```python
from build123d import *

# Parameters (mm, degrees)
F1_DEPTH = 3
F2_W     = 90
F2_H     = 55
F3_DEPTH = 24
F4_R     = 1.25
F5_DEPTH = 10
F6_W     = 13
F6_H     = 65
F7_DEPTH = 9
F8_R     = 3


with BuildPart() as f1:
    # F0 (on Top) → F1 (new body)
    with BuildSketch(Plane.XY):
        with BuildLine():
            ThreePointArc((0, 5), (1.464466, 1.464466), (5, 0))
            Line((5, 0), (99, 0))
            ThreePointArc((99, 0), (102.535534, 1.464466), (104, 5))
            Line((104, 5), (104, 60))
            ThreePointArc((104, 60), (102.535534, 63.535534), (99, 65))
            Line((99, 65), (5, 65))
            ThreePointArc((5, 65), (1.464466, 63.535534), (0, 60))
            Line((0, 60), (0, 5))
        make_face()
    extrude(amount=F1_DEPTH)

    # F2 (on face) → F3 (join)
    with BuildSketch(Plane.XY.offset(3)):
        with BuildLine():
            Line((0, 60), (0, 5))
            ThreePointArc((0, 5), (1.464466, 1.464466), (5, 0))
            Line((5, 0), (99, 0))
            ThreePointArc((99, 0), (102.535534, 1.464466), (104, 5))
            Line((104, 5), (104, 60))
            ThreePointArc((104, 60), (102.535534, 63.535534), (99, 65))
            Line((99, 65), (5, 65))
            ThreePointArc((5, 65), (1.464466, 63.535534), (0, 60))
        make_face()
        with Locations((52, 32.5)):
            Rectangle(F2_W, F2_H, mode=Mode.SUBTRACT)
    extrude(amount=F3_DEPTH)

    # F4 (on face) → F5 (cut)
    with BuildSketch(Plane.XY.offset(27)):
        with Locations((3.5, 10)):
            Circle(F4_R)
        with Locations((100.5, 55)):
            Circle(F4_R)
        with Locations((100.5, 10)):
            Circle(F4_R)
        with Locations((3.5, 55)):
            Circle(F4_R)
    extrude(amount=-F5_DEPTH, mode=Mode.SUBTRACT)

    # F6 (on face) → F7 (cut)
    with BuildSketch(Plane.XY.offset(27)):
        with Locations((19.5, 32.5)):
            Rectangle(F6_W, F6_H)
    extrude(amount=-F7_DEPTH, mode=Mode.SUBTRACT)

    # F8
    f8_edges = [f1.edges().sort_by_distance(p)[0] for p in [
        (26, 2.5, 18),
        (26, 62.5, 18),
        (13, 62.5, 18),
        (13, 2.5, 18),
    ]]
    fillet(f8_edges, radius=F8_R)


solid = f1.part
```
Part model, mm, in its own coordinate system. A direction names the side the tool comes from. Round coordinates to 2 decimals unless told otherwise and drop trailing zeros. Order: outer loops, then holes, each group sorted by start corner. A loop starts at its lowest first (then second) coordinate and runs counter-clockwise, first axis right, second up. Notation, with made-up numbers: M 44,-21 L 63,-21 A18 ccw 63,1 Z; hole C 53,47.25 d4. An arc over 180 degrees is marked long. Answer in a Markdown table with one row per item. Add a question column.
Q1. Cut at A-A on z = 7.25. Give the cut face in (x, y), and give its area (3 significant figures).
Q2. Wall check: L1, parallel to Y at x = 67, z = 17.5; L2, parallel to X at y = 54, z = 8; L3, parallel to Y at x = 100.5, z = 24. Give the ranges that are in metal, low to high. Write a range as from..to.
Q3. Cut at C-C on x = 88. Give the cut face in (y, z).
Q4. 3-axis set-ups, long thin cutter, end or side, ignore diameter. For faces 5 (the face through (101.69, 10.38, 22.07)), 6 (the face through (51, 0, 13)), 7 (the face through (19, 3, 18)): which of +Z, -Z, +X, -X, +Y, -Y reach the whole face in a straight line?
Q5. Cut at D-D on y = 55. Give the cut face in (x, z), and give its area (3 significant figures).
Q6. Cut at B-B on y = 20. Give the cut face in (x, z), and give its area (3 significant figures).
Q7. Pin check, flat tips, straight feed: pin 1 (2.5 mm diameter, centred on x = 21, y = 1.5, fed in from +Z); pin 2 (5 mm diameter, centred on x = 57, y = 42, fed in from +Z); pin 3 (1.5 mm diameter, centred on y = 1.5, z = 23.5, fed in from -X). Stop position of each tip, or through.
Q8. Mould opens along X. For faces 1 (the face through (7, 32, 15)), 2 (the face through (100, 55, 17)), 3 (the face through (102, 1, 13)), 4 (the face through (53, 65, 13)) say: +X half, -X half, draft (parallel to the pull), parting line (faces both ways), or undercut.
Established:
| question | item | result |
|---|---|---|
| 1 | outline | M 0,5 A5 ccw 5,0 L 99,0 A5 ccw 104,5 L 104,60 A5 ccw 99,65 L 5,65 A5 ccw 0,60 Z; hole M 7,5 L 97,5 L 97,60 L 7,60 Z |
| 1 | area | 1,790 mm2 |
| 2 | L1 | y = 0..5, 60..65 |
| 2 | L2 | x = 0..7, 97..104 |
| 2 | L3 | y = 0.23..8.75, 11.25..53.75, 56.25..64.77 |
| 3 | outline | M 0,0 L 65,0 L 65,27 L 60,27 L 60,3 L 5,3 L 5,27 L 0,27 Z |
| 4 | face 5 | +Z |
| 4 | face 6 | +Z, -Z, +X, -X, -Y |
| 4 | face 7 | +Z, +Y, -Y |
| 5 | outline | M 0,0 L 104,0 L 104,27 L 101.75,27 L 101.75,17 L 99.25,17 L 99.25,27 L 97,27 L 97,3 L 7,3 L 7,27 L 4.75,27 L 4.75,17 L 2.25,17 L 2.25,27 L 0,27 Z |
| 5 | area | 598 mm2 |
| 6 | outline | M 0,0 L 104,0 L 104,27 L 97,27 L 97,3 L 7,3 L 7,27 L 0,27 Z |
| 6 | area | 648 mm2 |
| 7 | pin 1 | stops at z = 18 |
| 7 | pin 2 | stops at z = 3 |
| 7 | pin 3 | stops at x = 0.82 |
| 8 | face 1 | undercut |
| 8 | face 2 | undercut |
| 8 | face 3 | +X half |
| 8 | face 4 | draft |
